from build123d import *

# Parameters (mm, degrees)
MODEL_R                  = 1.25
RESSALTO_EXTRUS_O1_DEPTH = 20


with BuildPart() as part:
    # Model → Ressalto-extrusão1 (new body)
    with BuildSketch(Plane.XY):
        with BuildLine():
            Line((11.694931393, 184.007671687), (18.798816999, 196.310732401))
            ThreePointArc((18.798816999, 196.310732401), (20.628779754, 198.140639612), (23.128489927, 198.81054493))
            Line((23.128489927, 198.81054493), (104.854461984, 198.816198006))
            ThreePointArc((104.854461984, 198.816198006), (107.353091528, 198.147315496), (109.183125054, 196.319330074))
            Line((109.183125054, 196.319330074), (116.309159239, 183.99727285))
            ThreePointArc((116.309159239, 183.99727285), (116.980841789, 181.495674545), (116.310694096, 178.993664633))
            Line((116.310694096, 178.993664633), (75.435169171, 108.213155276))
            ThreePointArc((75.435169171, 108.213155276), (73.605079007, 106.383366964), (71.105317099, 105.713631437))
            Line((71.105317099, 105.713631437), (56.87911326, 105.713631437))
            ThreePointArc((56.87911326, 105.713631437), (54.378684602, 106.383751932), (52.548491341, 108.214488825))
            Line((52.548491341, 108.214488825), (11.694328258, 179.008341616))
            ThreePointArc((11.694328258, 179.008341616), (11.024950213, 181.508087444), (11.694931393, 184.007671687))
        make_face()
        with Locations((23.321458454, 185.48579228)):
            Circle(MODEL_R, mode=Mode.SUBTRACT)
        with Locations((63.991701896, 114.980441868)):
            Circle(MODEL_R, mode=Mode.SUBTRACT)
        with Locations((104.686697162, 185.492130263)):
            Circle(MODEL_R, mode=Mode.SUBTRACT)
        with BuildLine():
            Line((30.926807018, 178.651666079), (33.041188625, 182.313516329))
            ThreePointArc((33.041188625, 182.313516329), (34.870788611, 184.143214068), (37.370023748, 184.813328729))
            Line((37.370023748, 184.813328729), (90.685321042, 184.825950173))
            ThreePointArc((90.685321042, 184.825950173), (93.184425519, 184.157277084), (95.014821917, 182.329082369))
            Line((95.014821917, 182.329082369), (97.129519324, 178.672431029))
            ThreePointArc((97.129519324, 178.672431029), (97.801202073, 176.169904784), (97.130125767, 173.667215847))
            Line((97.130125767, 173.667215847), (70.44074248, 127.491170956))
            ThreePointArc((70.44074248, 127.491170956), (68.610777042, 125.662525758), (66.111818822, 124.993254082))
            Line((66.111818822, 124.993254082), (61.884877937, 124.993254082))
            ThreePointArc((61.884877937, 124.993254082), (59.3841246, 125.66356209), (57.553881257, 127.494760984))
            Line((57.553881257, 127.494760984), (30.925829122, 173.652985522))
            ThreePointArc((30.925829122, 173.652985522), (30.256825897, 176.152456774), (30.926807018, 178.651666079))
        make_face(mode=Mode.SUBTRACT)
    extrude(amount=RESSALTO_EXTRUS_O1_DEPTH)


solid = part.part
Could you check a few things on this model? Use its own coordinates, in mm. A direction names the side the tool comes from. Give positions to 0.01 mm unless a question says otherwise; leave off trailing zeros. Order: outer loops, then holes, each group sorted by start corner. A loop starts at its lowest first (then second) coordinate and runs counter-clockwise, first axis right, second up.
Item 1: I need wall thicknesses on line 1 (Y direction, x = 94, z = 3.75); line 2 (Y direction, x = 90, z = 8.25); line 3 (X direction, y = 176, z = 17.25). Which ranges of each line are inside material? Lowest first, please.
Item 2: If we mould it in two halves opening along X, with no side actions, what happens to faces 1 (the face through (96.16, 144.1, 9.86)), 2 (the face through (41, 153, 20)), 3 (the face through (23.159, 186.725, 9.86))? For each: pulls with the +X half, pulls with the -X half, needs draft (parallel to the pull), parting line crosses it, or undercut.
Item 3: If we section it at C-C, the plane x = 68.5: Write out the boundary of the cut face in (y, z).
Item 4: If we section it at D-D, the plane y = 112: Write out the boundary of the cut face in (x, z).
Item 5: For faces 4 (the face through (44.4, 150.3, 9.9)), 5 (the face through (11.025, 181.471, 9.86)), which set-ups out of +Z, -Z, +X, -X, +Y, -Y let a thin tool reach every point of the face, with its end or its side?
Item 6: I'm going to push flat-ended pins straight in: pin 1 (3 mm diameter, centred on x = 67, z = 8.5, fed in from +Y); pin 2 (2 mm diameter, centred on x = 104.69, y = 185.49, fed in from -Z); pin 3 (6 mm diameter, centred on y = 151.5, z = 6.5, fed in from +X). Where does each tip first touch, or does it pass through?
Item 7: If we section it at A-A, the plane y = 153: Write out the boundary of the cut face in (x, z), plus the area to 3 significant figures.
Item 8: If we section it at B-B, the plane z = 8: Write out the boundary of the cut face in (x, y), plus the area to 3 significant figures.
Values:
1. line 1: y = 140.36 to 168.25, 183.57 to 198.82
1. line 2: y = 133.43 to 161.33, 184.83 to 198.82
1. line 3: x = 13.43 to 30.26, 97.8 to 114.58
2. face 1: pulls with the +X half
2. face 2: needs draft
2. face 3: undercut
3. outline: (105.71, 0) - (125.6, 0) - (125.6, 20) - (105.71, 20) - close; (184.82, 0) - (198.81, 0) - (198.81, 20) - (184.82, 20) - close
4. outline: (50.36, 0) - (77.62, 0) - (77.62, 20) - (50.36, 20) - close
5. face 4: +Z, -Z
5. face 5: +Z, -Z, -X
6. pin 1: stops at y = 198.81
6. pin 2: passes through
6. pin 3: stops at x = 102.17
7. outline: (26.7, 0) - (42.84, 0) - (42.84, 20) - (26.7, 20) - close; (85.18, 0) - (101.3, 0) - (101.3, 20) - (85.18, 20) - close
7. area: 645 mm2
8. outline: (11.69, 179.01) - (52.55, 108.21) arc R5 ccw to (56.88, 105.71) - (71.11, 105.71) arc R5 ccw to (75.44, 108.21) - (116.31, 178.99) arc R5 ccw to (116.31, 184) - (109.18, 196.32) arc R5 ccw to (104.85, 198.82) - (23.13, 198.81) arc R5 ccw to (18.8, 196.31) - (11.69, 184.01) arc R5 ccw to start; hole circle Ø2.5 at (23.32, 185.49); hole (30.93, 173.65) - (57.55, 127.49) arc R5 ccw to (61.88, 124.99) - (66.11, 124.99) arc R5 ccw to (70.44, 127.49) - (97.13, 173.67) arc R5 ccw to (97.13, 178.67) - (95.01, 182.33) arc R5 ccw to (90.69, 184.83) - (37.37, 184.81) arc R5 ccw to (33.04, 182.31) - (30.93, 178.65) arc R5 ccw to start; hole circle Ø2.5 at (63.99, 114.98); hole circle Ø2.5 at (104.69, 185.49)
8. area: 3,930 mm2
